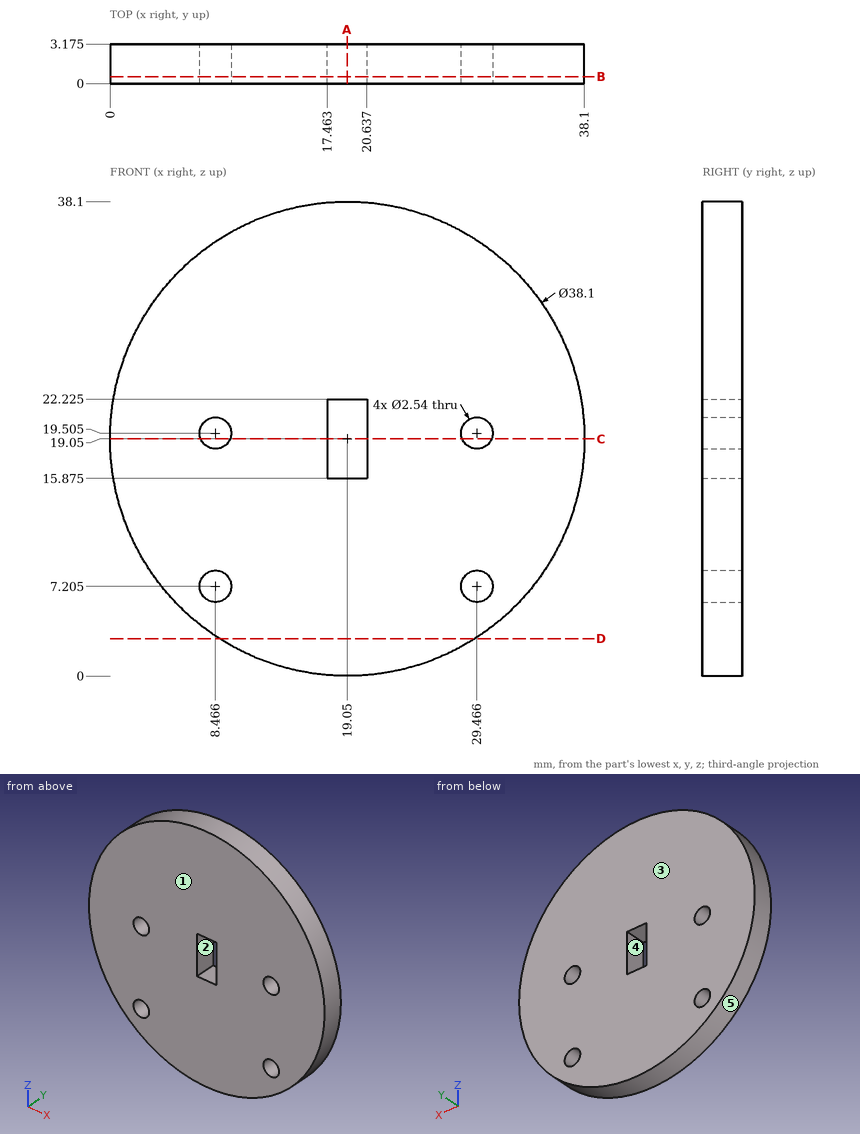
Job drawing, mm, ordinate dimensions from the low corner. One solid piece. A direction names the side the tool comes from. Coordinates: 2 decimals unless noted, no trailing zeros. Write each loop counter-clockwise with the first axis right and the second up, starting at its lowest first coordinate (ties: lowest second). Pieces come first, ordered by that corner, then holes.
Item 1: Which spindle directions (+Z, -Z, +X, -X, +Y, -Y) get a long thin tool onto all of the face, cutting with end or side? Do the marked faces 1 and 2. Say none if no direction does.
Item 2: Slice it at A-A (x = 19.05). Write the cut outline in (y, z) (1 decimal), and give its area (3 significant figures).
Item 3: Pin check, flat tips, straight feed: pin 1 (3 mm diameter, centred on x = 29.47, z = 7.2, fed in from +Y) (1 decimal); pin 2 (1.6 mm diameter, centred on y = 1.5, z = 20, fed in from -X); pin 3 (1 mm diameter, centred on x = 18, y = 2, fed in from -Z); pin 4 (1.5 mm diameter, centred on x = 23, y = 2, fed in from +Z). Stop position of each tip, or through.
Item 4: Slice it at B-B (y = 0.55). Count the separate pieces of the cut face and the enclosed holes in it, and give its area (3 significant figures).
Item 5: Mould opens along X. For the marked faces 3, 4 and 5 say: released by +X, released by -X, zero draft, split by the parting line, or undercut.
Item 6: Probe line 1 (X direction, y = 2.15, z = 19.5) (1 decimal); line 2 (Z direction, x = 9.5, y = 0.9) (1 decimal); line 3 (X direction, y = 0.25, z = 20) (1 decimal). List the from-to ranges inside material, lowest first.
Item 7: Slice it at D-D (z = 3). Write the cut outline in (x, y) (1 decimal).
Item 8: Slice it at C-C (z = 19.05). Write the cut outline in (x, y) (1 decimal).
Results found:
1. face 1: +Z, -Z, +X, -X, -Y
1. face 2: +Y, -Y
2. outline: (0, 0) - (3.2, 0) - (3.2, 15.9) - (0, 15.9) - close; (0, 22.2) - (3.2, 22.2) - (3.2, 38.1) - (0, 38.1) - close
2. area: 101 mm2
3. pin 1: stops at y = 3.2
3. pin 2: stops at x = 0
3. pin 3: stops at z = 0.01
3. pin 4: stops at z = 37.83
4. separate pieces: 1
4. enclosed holes: 5
4. area: 1,100 mm2
5. face 3: zero draft
5. face 4: undercut
5. face 5: split by the parting line
6. line 1: x = 0 to 7.2, 9.7 to 17.5, 20.6 to 28.2, 30.7 to 38.1
6. line 2: z = 2.6 to 6.5, 7.9 to 18.8, 20.2 to 35.5
6. line 3: x = 0 to 7.3, 9.6 to 17.5, 20.6 to 28.3, 30.6 to 38.1
7. outline: (8.8, 0) - (29.3, 0) - (29.3, 3.2) - (8.8, 3.2) - close
8. outline: (0, 0) - (7.3, 0) - (7.3, 3.2) - (0, 3.2) - close; (9.7, 0) - (17.5, 0) - (17.5, 3.2) - (9.7, 3.2) - close; (20.6, 0) - (28.3, 0) - (28.3, 3.2) - (20.6, 3.2) - close; (30.7, 0) - (38.1, 0) - (38.1, 3.2) - (30.7, 3.2) - close
